```python
from build123d import *

# Parameters (mm, degrees)
EXTRUDE_START    = 4
SKETCH_1_R       = 3.8
SKETCH_1_R_2     = 1.55
SKETCH_1_R_3     = 1.553894019
EXTRUDE_7_DEPTH  = 1
EXTRUDE_START_2  = -4
SKETCH_6_R       = 3.8
SKETCH_6_R_2     = 1.7
SKETCH_6_R_3     = 1.55
SKETCH_6_R_4     = 1.703894019
SKETCH_6_R_5     = 1.553894019
EXTRUDE_11_DEPTH = 1
SKETCH_4_R       = 1.55
EXTRUDE_12_DEPTH = 5.25
SKETCH_4_5_R     = 1.55
SKETCH_4_5_R_2   = 1.553894019
EXTRUDE_13_DEPTH = 5.25


with BuildPart() as part:
    # Sketch 1 → Extrude 7 (new body)
    # profile 1 of 3: a face of its own
    with BuildSketch(Plane(origin=(0, 0, 0), x_dir=(1, 0, 0), z_dir=(0, 1, 0)).offset(EXTRUDE_START)):
        with Locations((-56.235722287, 24.732868077)):
            Circle(SKETCH_1_R)
        with Locations(Location((-56.235722287, 24.732868077, 0), (0, 0, 270))):
            Circle(SKETCH_1_R_2, mode=Mode.SUBTRACT)
    # profile 2 of 3: a face of its own
    with BuildSketch(Plane(origin=(0, 0, 0), x_dir=(1, 0, 0), z_dir=(0, 1, 0)).offset(EXTRUDE_START)):
        with BuildLine():
            ThreePointArc((-56.093079937, 28.530189917), (-53.498749422, 27.368959792), (-52.435722287, 24.732868077))
            ThreePointArc((-52.435722287, 24.732868077), (-53.548716519, 22.045862308), (-56.235722287, 20.932868077))
            add(Edge.make_bspline(
                [(-56.235722287, 20.932868077), (-54.105831048, 20.932868077), (-49.896032342, 22.477788173), (-46.252423284, 20.705707547), (-43.855722287, 20.705707547)],
                knots=[0, 0, 0, 0, 0.498510271, 1, 1, 1, 1], degree=3))
            ThreePointArc((-43.855722287, 20.705707547), (-47.655142775, 24.572069864), (-43.723017894, 28.303389675))
            add(Edge.make_bspline(
                [(-56.093079937, 28.530189917), (-53.942583983, 28.449408827), (-49.768599584, 26.149491118), (-46.433977381, 28.398120151), (-43.723017894, 28.303389675)],
                knots=[0, 0, 0, 0, 0.490575379, 1, 1, 1, 1], degree=3))
        make_face()
    # profile 3 of 3: a face of its own
    with BuildSketch(Plane(origin=(0, 0, 0), x_dir=(1, 0, 0), z_dir=(0, 1, 0)).offset(EXTRUDE_START)):
        with Locations((-43.855722287, 24.505707547)):
            Circle(SKETCH_1_R)
        with Locations(Location((-43.855722287, 24.505707547, 0), (0, 0, 270))):
            Circle(SKETCH_1_R_3, mode=Mode.SUBTRACT)
    extrude(amount=EXTRUDE_7_DEPTH)



with BuildPart() as body_2:
    # Sketch 6 → Extrude 11 (new body)
    # profile 1 of 5: a face of its own
    with BuildSketch(Plane(origin=(0, 0, 0), x_dir=(1, 0, 0), z_dir=(0, 1, 0)).offset(EXTRUDE_START_2)):
        with BuildLine():
            ThreePointArc((-43.855722287, 20.705707547), (-47.655142775, 24.572069864), (-43.723017894, 28.303389675))
            add(Edge.make_bspline(
                [(-56.093079937, 28.530189917), (-53.942583983, 28.449408827), (-49.768599584, 26.149491118), (-46.433977381, 28.398120151), (-43.723017894, 28.303389675)],
                knots=[0, 0, 0, 0, 0.490575379, 1, 1, 1, 1], degree=3))
            ThreePointArc((-56.093079937, 28.530189917), (-53.498749422, 27.368959792), (-52.435722287, 24.732868077))
            ThreePointArc((-52.435722287, 24.732868077), (-53.548716519, 22.045862308), (-56.235722287, 20.932868077))
            add(Edge.make_bspline(
                [(-56.235722287, 20.932868077), (-54.105831048, 20.932868077), (-49.896032342, 22.477788173), (-46.252423284, 20.705707547), (-43.855722287, 20.705707547)],
                knots=[0, 0, 0, 0, 0.498510271, 1, 1, 1, 1], degree=3))
        make_face()
    # profile 2 of 5: a face of its own
    with BuildSketch(Plane(origin=(0, 0, 0), x_dir=(1, 0, 0), z_dir=(0, 1, 0)).offset(EXTRUDE_START_2)):
        with Locations((-56.235722287, 24.732868077)):
            Circle(SKETCH_6_R)
        with Locations((-56.235722287, 24.732868077)):
            Circle(SKETCH_6_R_2, mode=Mode.SUBTRACT)
    # profile 3 of 5: a face of its own
    with BuildSketch(Plane(origin=(0, 0, 0), x_dir=(1, 0, 0), z_dir=(0, 1, 0)).offset(EXTRUDE_START_2)):
        with Locations((-56.235722287, 24.732868077)):
            Circle(SKETCH_6_R_2)
        with Locations(Location((-56.235722287, 24.732868077, 0), (0, 0, 270))):
            Circle(SKETCH_6_R_3, mode=Mode.SUBTRACT)
    # profile 4 of 5: a face of its own
    with BuildSketch(Plane(origin=(0, 0, 0), x_dir=(1, 0, 0), z_dir=(0, 1, 0)).offset(EXTRUDE_START_2)):
        with Locations((-43.855722287, 24.505707547)):
            Circle(SKETCH_6_R)
        with Locations((-43.855722287, 24.505707547)):
            Circle(SKETCH_6_R_4, mode=Mode.SUBTRACT)
    # profile 5 of 5: a face of its own
    with BuildSketch(Plane(origin=(0, 0, 0), x_dir=(1, 0, 0), z_dir=(0, 1, 0)).offset(EXTRUDE_START_2)):
        with Locations((-43.855722287, 24.505707547)):
            Circle(SKETCH_6_R_4)
        with Locations(Location((-43.855722287, 24.505707547, 0), (0, 0, 270))):
            Circle(SKETCH_6_R_5, mode=Mode.SUBTRACT)
    extrude(amount=-EXTRUDE_11_DEPTH)


with BuildPart() as part_1:
    add(part.part)

    add(body_2.part)  # Extrude 12 merges body 2
    # Sketch 4 → Extrude 12 (add, symmetric)
    with BuildSketch(Plane(origin=(0, 0, 0), x_dir=(1, 0, 0), z_dir=(0, 1, 0))):
        with Locations(Location((-56.235722287, 24.732868077, 0), (0, 0, 90))):
            Circle(SKETCH_4_R)
    extrude(amount=EXTRUDE_12_DEPTH, both=True)

    # Sketch 4_5 → Extrude 13 (add, symmetric)
    with BuildSketch(Plane(origin=(0, 0, 0), x_dir=(1, 0, 0), z_dir=(0, 1, 0))):
        with Locations(Location((-56.235722287, 24.732868077, 0), (0, 0, 90))):
            Circle(SKETCH_4_5_R)
        with Locations(Location((-43.855722287, 24.505707547, 0), (0, 0, 90))):
            Circle(SKETCH_4_5_R_2)
    extrude(amount=EXTRUDE_13_DEPTH, both=True)


solid = part_1.part
```
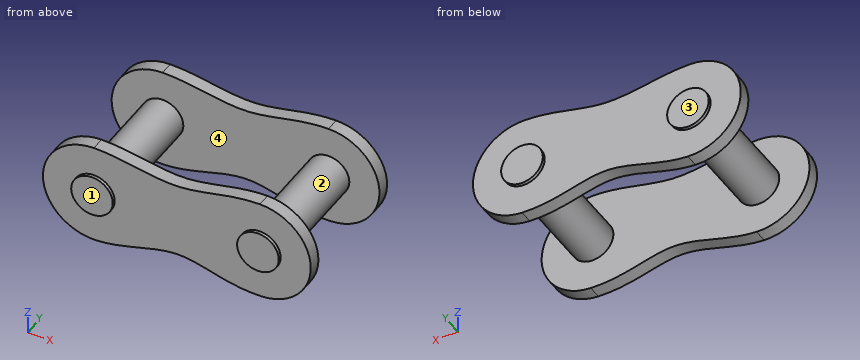
Verification items for the finished model (mm, model axes). Face numbers are marked on the shaded views. A direction names the side the tool comes from. Coordinates: 2 decimals unless noted, no trailing zeros. Order: outer loops, then holes, each group sorted by start corner. A loop starts at its lowest first (then second) coordinate and runs counter-clockwise, first axis right, second up. Notation, with made-up numbers: (-23.75, 38.25) -> (19.25, 38.25) arc R9 ccw to (19.25, 48.25) -> close; hole circle Ø5 at (-4.75, 63). An arc over 180 degrees is marked (long way). Answer as CSV lines item,"result". Start each with the question number.
1) Cross-section at C-C, the plane x = -42. Record the boundary of the cut face in (y, z).
2) Cross-section at A-A, the plane z = -22.25. Record the boundary of the cut face in (x, y).
3) Release check for a two-part mould opening along X. For the marked faces 3 and 4 record: released by +X, released by -X, zero draft, split by the parting line, or undercut.
4) Set-up check for the marked faces 1 and 2: record each of +Z, -Z, +X, -X, +Y, -Y from which the full face is reachable in a straight line by a thin tool's end or side.
5) Cross-section at B-B, the plane y = -0.5. Record the boundary of the cut face in (x, z).
6) Material ranges on L1, parallel to Y at x = -45.5, z = -21.5; L2, parallel to X at y = 1.75, z = -23.75; L3, parallel to X at y = -3.25, z = -25.5, recorded low to high. Write a range as [from, to].
7) Gauge pin test, flat ends, axial feed: pin 1 Ø1 at (x, y) = (-44, -3) entering from -Z; pin 2 Ø1.5 at (x, y) = (-44.5, 0.5) entering from +Z; pin 3 Ø4 at (x, z) = (-46.5, -23) entering from -Y. Record the tip position at first contact, or that the pin passes through.
Conclusion:
1,outline,"(-5, -27.82) -> (-4, -27.82) -> (-4, -21.19) -> (-5, -21.19) -> close; (4, -27.82) -> (5, -27.82) -> (5, -21.19) -> (4, -21.19) -> close"
2,outline,"(-59.11, -5) -> (-40.8, -5) -> (-40.8, -4) -> (-59.11, -4) -> close; (-59.11, 4) -> (-40.8, 4) -> (-40.8, 5) -> (-59.11, 5) -> close"
3,face 3,"zero draft"
3,face 4,"undercut"
4,face 1,"+Z, -Z, +X, -X, -Y"
4,face 2,"none"
5,outline,"circle Ø3.1 at (-56.24, -24.73); circle Ø3.11 at (-43.86, -24.51)"
6,L1,"y = [-5, -4], [4, 5]"
6,L2,"x = [-57.43, -55.04], [-45.21, -42.5]"
6,L3,"x = [-57.58, -54.89], [-45.05, -42.66]"
7,pin 1,"stops at z = -26.06"
7,pin 2,"stops at z = -22.95"
7,pin 3,"stops at y = -5.25"
